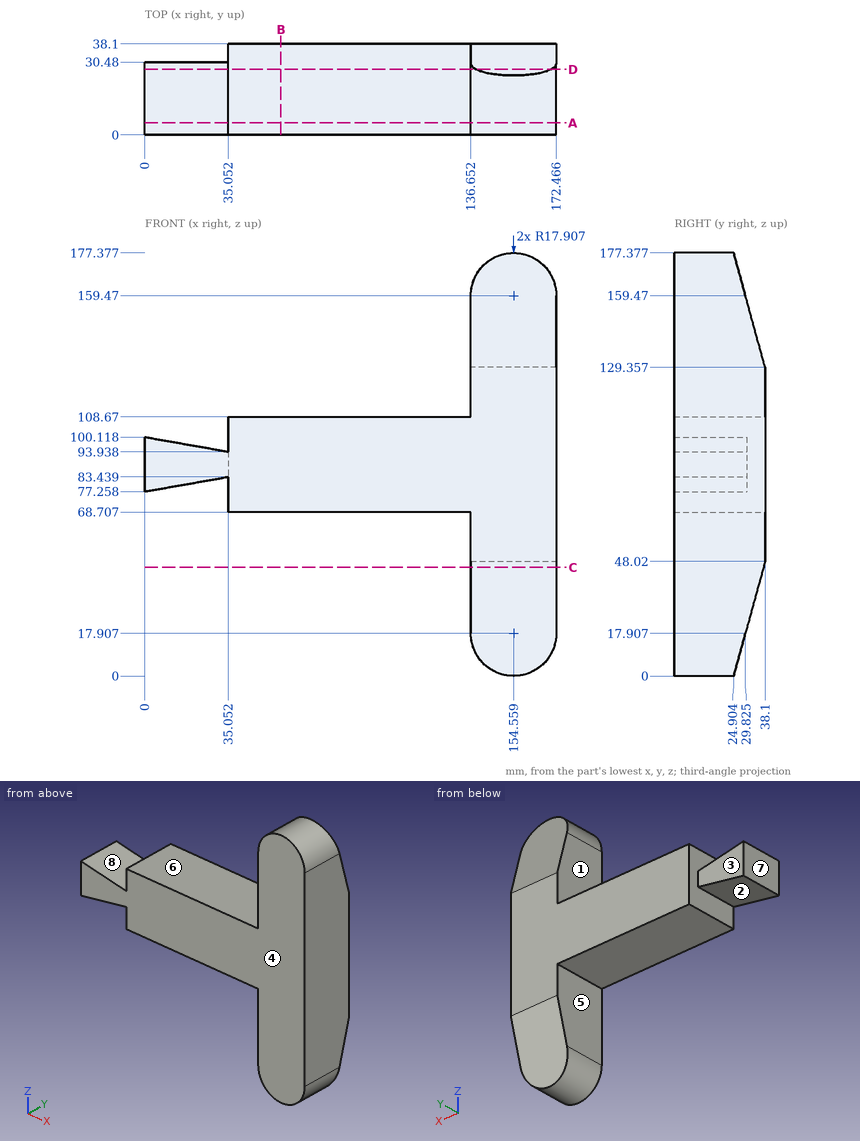
Input: dimensioned drawing with shaded views. Units: mm. Origin: part minimum x, y, z. A direction names the side the tool comes from. Give positions to 0.01 mm unless a question says otherwise; leave off trailing zeros. Order: outer loops, then holes, each group sorted by start corner. A loop starts at its lowest first (then second) coordinate and runs counter-clockwise, first axis right, second up. Notation, with made-up numbers: (76, 15) -> (125, 15) arc R26 ccw to (125, 46) -> close; hole circle Ø5 at (88.25, 7). An arc over 180 degrees is marked (long way). Use one line per item in the form item = value.
1) Section B-B, the plane x = 57. Return loops of the section in (y, z), and give its area (3 significant figures).
Response values:
outline = (0, 68.71) -> (38.1, 68.71) -> (38.1, 108.67) -> (0, 108.67) -> close
area = 1,520 mm^2
2) Mould query, pull axis X, two halves, no side actions, for the marked faces 1, 2 and 3. Classes: pulls with the +X half, pulls with the -X half, needs draft (parallel to the pull), parting line crosses it, or undercut.
Response values:
face_1 = pulls with the -X half
face_2 = undercut
face_3 = needs draft
3) Line query: probe 1 along X at (y, z) = (5, 52); probe 2 along X at (y, z) = (8.5, 107.5); probe 3 along Z at (x, y) = (72, 8). Output: solid intervals per line, ascending.
Response values:
probe_1 = 136.65 to 172.47
probe_2 = 35.05 to 172.47
probe_3 = 68.71 to 108.67
4) Section A-A, the plane y = 5. Return loops of the section in (x, z), and give its area (3 significant figures).
Response values:
outline = (0, 77.26) -> (35.05, 83.44) -> (35.05, 68.71) -> (136.65, 68.71) -> (136.65, 17.91) arc R17.91 ccw to (172.47, 17.91) -> (172.47, 159.47) arc R17.91 ccw to (136.65, 159.47) -> (136.65, 108.67) -> (35.05, 108.67) -> (35.05, 93.94) -> (0, 100.12) -> close
area = 10,700 mm^2
5) Section C-C, the plane z = 45.5. Return loops of the section in (x, y), and give its area (3 significant figures).
Response values:
outline = (136.65, 0) -> (172.47, 0) -> (172.47, 37.41) -> (136.65, 37.41) -> close
area = 1,340 mm^2
6) Section D-D, the plane y = 27.5. Return loops of the section in (x, z).
Response values:
outline = (0, 77.26) -> (35.05, 83.44) -> (35.05, 68.71) -> (136.65, 68.71) -> (136.65, 17.91) arc R17.91 ccw to (138.78, 9.45) -> (170.34, 9.45) arc R17.91 ccw to (172.47, 17.91) -> (172.47, 159.47) arc R17.91 ccw to (170.34, 167.93) -> (138.78, 167.93) arc R17.91 ccw to (136.65, 159.47) -> (136.65, 108.67) -> (35.05, 108.67) -> (35.05, 93.94) -> (0, 100.12) -> close
7) Reachability of the marked faces 4, 5, 6, 7 and 8 from +Z, -Z, +X, -X, +Y, -Y: full face, straight path, thin tool, end or side. Return the list, or none.
Response values:
face_4 = +Z, -Z, +X, -X, -Y
face_5 = -Z, -X, +Y, -Y
face_6 = +Z, -X, +Y, -Y
face_7 = +Z, -Z, -X, +Y, -Y
face_8 = +Z, +Y, -Y
8) First-contact query: pin 1 Ø1.5 at (x, y) = (46.5, 6) entering from +Z; pin 2 Ø11.5 at (x, z) = (26.5, 91) entering from +Y; pin 3 Ø11.5 at (x, y) = (77, 15.5) entering from -Z. Flat tips, straight axial feed; report the tip coordinate or a pass-through.
Response values:
pin_1 = 108.67
pin_2 = 30.48
pin_3 = 68.71
